Input: part model. Units: mm. Frame: model coordinates. Face numbers are marked on the shaded views. A direction names the side the tool comes from. Round coordinates to 2 decimals unless told otherwise and drop trailing zeros. Order: outer loops, then holes, each group sorted by start corner. A loop starts at its lowest first (then second) coordinate and runs counter-clockwise, first axis right, second up.
Item 1: Cut plane D-D on z = 7. Output: boundary loops of the cut face in (x, y).
Item 2: Reachability of the marked faces 1, 2 and 3 from +Z, -Z, +X, -X, +Y, -Y: full face, straight path, thin tool, end or side. Return the list, or none.
Item 3: Cut plane A-A on y = 0. Output: boundary loops of the cut face in (x, z).
Item 4: Line query: L1, parallel to Y at x = -7.75, z = -1.7; L2, parallel to Z at x = 5, y = 1; L3, parallel to Z at x = 11.5, y = 14. Output: solid intervals per line, ascending.
Item 5: First-contact query: pin 1 (2 mm diameter, centred on y = -11.5, z = -39.5, fed in from -X); pin 2 (1 mm diameter, centred on x = 8, y = 13.5, fed in from +Z); pin 3 (5 mm diameter, centred on x = -14, y = -5.5, fed in from +Z). Flat tips, straight axial feed; report the tip coordinate or a pass-through.
Item 6: Cut plane B-B on z = -29. Output: boundary loops of the cut face in (x, y), then the cut area to 3 significant figures.
Item 7: Cut plane C-C on x = -7.75. Output: boundary loops of the cut face in (y, z).
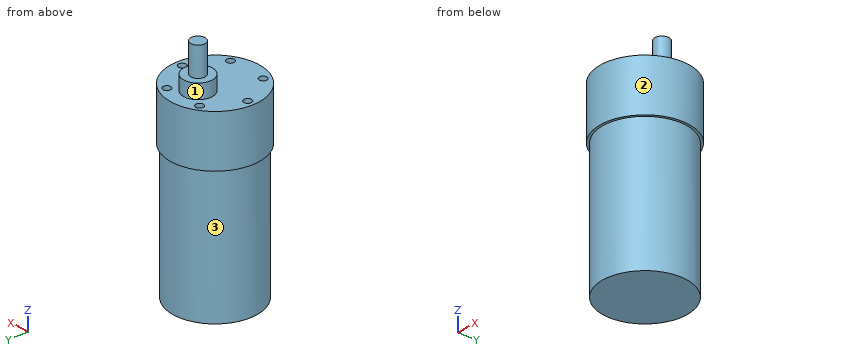
```python
from build123d import *

# Parameters (mm, degrees)
ESBO_O1_R                = 18.5
RESSALTO_EXTRUS_O1_DEPTH = 21.5
ESBO_O2_R                = 17.5
RESSALTO_EXTRUS_O2_DEPTH = 55.5
ESBO_O5_R                = 6
RESSALTO_EXTRUS_O6_DEPTH = 6
ESBO_O6_R                = 3
RESSALTO_EXTRUS_O7_DEPTH = 12
ESBO_O7_R                = 1.6
CORTE_EXTRUS_O1_DEPTH    = 6


with BuildPart() as part:
    # Esboço1 → Ressalto-extrusão1 (new body)
    with BuildSketch(Plane.XY):
        Circle(ESBO_O1_R)
    extrude(amount=-RESSALTO_EXTRUS_O1_DEPTH)

    # Esboço2 → Ressalto-extrusão2 (add)
    with BuildSketch(Plane(origin=(0, 0, -21.5), x_dir=(-1, 0, 0), z_dir=(0, 0, -1))):
        Circle(ESBO_O2_R)
    extrude(amount=RESSALTO_EXTRUS_O2_DEPTH)

    # Esboço5 → Ressalto-extrusão6 (add)
    with BuildSketch(Plane.XY):
        with Locations((0, 7.2)):
            Circle(ESBO_O5_R)
    extrude(amount=RESSALTO_EXTRUS_O6_DEPTH)

    # Esboço6 → Ressalto-extrusão7 (add)
    with BuildSketch(Plane.XY.offset(6)):
        with Locations((0, 7.2)):
            Circle(ESBO_O6_R)
    extrude(amount=RESSALTO_EXTRUS_O7_DEPTH)

    # Esboço7 → Corte-extrusão1 (cut)
    with BuildSketch(Plane.XY):
        with Locations((-7.75, 13.423393759)):
            Circle(ESBO_O7_R)
        with Locations((7.75, 13.423393759)):
            Circle(ESBO_O7_R)
        with Locations((15.5, 0)):
            Circle(ESBO_O7_R)
        with Locations((7.75, -13.423393759)):
            Circle(ESBO_O7_R)
        with Locations((-7.75, -13.423393759)):
            Circle(ESBO_O7_R)
        with Locations((-15.5, 0)):
            Circle(ESBO_O7_R)
    extrude(amount=-CORTE_EXTRUS_O1_DEPTH, mode=Mode.SUBTRACT)


solid = part.part
```
From the geometry:
1. outline: circle Ø6 at (0, 7.2)
2. face 1: +Z
2. face 2: +Z, -Z
2. face 3: -Z
3. outline: (-18.5, -21.5) - (-17.5, -21.5) - (-17.5, -77) - (17.5, -77) - (17.5, -21.5) - (18.5, -21.5) - (18.5, 0) - (17.1, 0) - (17.1, -6) - (13.9, -6) - (13.9, 0) - (-13.9, 0) - (-13.9, -6) - (-17.1, -6) - (-17.1, 0) - (-18.5, 0) - close
4. L1: y = -16.8 to -15.02, -11.82 to 11.82, 15.02 to 16.8
4. L2: z = -77 to 0
4. L3: z = -21.5 to 0
5. pin 1: stops at x = -14
5. pin 2: stops at z = -6
5. pin 3: stops at z = 0
6. outline: circle Ø35 at (0, 0)
6. area: 962 mm2
7. outline: (-16.8, -21.5) - (-15.69, -21.5) - (-15.69, -77) - (15.69, -77) - (15.69, -21.5) - (16.8, -21.5) - (16.8, 0) - (15.02, 0) - (15.02, -6) - (11.82, -6) - (11.82, 0) - (-11.82, 0) - (-11.82, -6) - (-15.02, -6) - (-15.02, 0) - (-16.8, 0) - close
